Source: CAD feature listing. Evaluate the final solid. Frame: model axes, mm. A direction names the side the tool comes from. Give positions to 0.01 mm unless a question says otherwise; leave off trailing zeros. Order: outer loops, then holes, each group sorted by start corner. A loop starts at its lowest first (then second) coordinate and runs counter-clockwise, first axis right, second up. Notation, with made-up numbers: M 58.25,-17.75 L 89.25,-17.75 A19 cw 89.25,11.25 Z; hole C 34.5,26 d6. An arc over 180 degrees is marked long. Answer as a JSON object with one key per item and string values. Group by question number.
1. Material intervals for L1, parallel to Y at x = 0, z = 1.25; L2, parallel to X at y = -3.5, z = 1.25; L3, parallel to X at y = -16, z = 0.75, sorted ascending. Write a range as [from, to].
2. Section query B-B (y = 0). Output: boundary loops of the cut face in (x, z), plus the area to 3 significant figures.
3. Pull-direction query (Y, two-part tool) for faces 1 (the flat face through (15, 0, 2)), 2 (the cylindrical face through (-1.08, -4.88, 2.03)), 3 (the flat face through (-11, -15, 2)), 4 (the flat face through (11, 15, 2)); classes: +Y half, -Y half, draft (parallel to the pull), parting line (faces both ways), or undercut.
4. Section query C-C (z = 3). Output: boundary loops of the cut face in (x, y).
5. Section query A-A (x = 0). Output: boundary loops of the cut face in (y, z), plus the area to 3 significant figures.
6. Section query D-D (y = 15.5). Output: boundary loops of the cut face in (x, z).
7. Pin query (flat end, axial travel): P1, Ø1.2, axis at y = -16.5, z = 1, coming from the -X side; P2, Ø2, axis at x = 10, z = 1.5, coming from the +Y side; P3, Ø1.2, axis at x = -10.5, z = 1, coming from the -Y side; P4, Ø1, axis at x = -3.5, y = 2, coming from the -Z side. Return the tip coordinate at first contact, or that it passes through.
8. Set-up query: faces 5 (the flat face through (-7.5, 18, 2)), 6 (the flat face through (11, -15, 2)), 7 (the flat face through (7.5, 17, 2)). Return all of +Z, -Z, +X, -X, +Y, -Y with unobstructed straight access to the full face (end or side cutting, diameter ignored); none if empty.
from build123d import *

# Parameters (mm, degrees)
BOSS_EXTRUDE1_DEPTH = 4
SKETCH2_R           = 5
CUT_EXTRUDE1_DEPTH  = 4


with BuildPart() as part:
    # Sketch1 → Boss-Extrude1 (new body)
    with BuildSketch(Plane.XY):
        Polygon((-7.5, 15), (-15, 15), (-15, -15), (-7.5, -15), (-7.5, -20), (7.5, -20), (7.5, -15), (15, -15), (15, 15), (7.5, 15), (7.5, 20), (-7.5, 20), align=None)
    extrude(amount=BOSS_EXTRUDE1_DEPTH)

    # Sketch2 → Cut-Extrude1 (cut)
    with BuildSketch(Plane.XY.offset(4)):
        Circle(SKETCH2_R)
    extrude(amount=-CUT_EXTRUDE1_DEPTH, mode=Mode.SUBTRACT)


solid = part.part
Answer sheet:
{
 "1": {"L1": "[-20, -5], [5, 20]", "L2": "[-15, -3.57], [3.57, 15]", "L3": "[-7.5, 7.5]"},
 "2": {"outline": "M -15,0 L -5,0 L -5,4 L -15,4 Z; M 5,0 L 15,0 L 15,4 L 5,4 Z", "area": "80.0 mm^2"},
 "3": {"face 1": "draft", "face 2": "undercut", "face 3": "-Y half", "face 4": "+Y half"},
 "4": {"outline": "M -15,-15 L -7.5,-15 L -7.5,-20 L 7.5,-20 L 7.5,-15 L 15,-15 L 15,15 L 7.5,15 L 7.5,20 L -7.5,20 L -7.5,15 L -15,15 Z; hole C 0,0 d10"},
 "5": {"outline": "M -20,0 L -5,0 L -5,4 L -20,4 Z; M 5,0 L 20,0 L 20,4 L 5,4 Z", "area": "120 mm^2"},
 "6": {"outline": "M -7.5,0 L 7.5,0 L 7.5,4 L -7.5,4 Z"},
 "7": {"P1": "x = -7.5", "P2": "y = 15", "P3": "y = -15", "P4": "through"},
 "8": {"face 5": "+Z, -Z, -X, +Y", "face 6": "+Z, -Z, +X, -Y", "face 7": "+Z, -Z, +X, +Y"}
}
